Could you check a few things on this drawing? It's one solid part, dimensions in mm from its lowest x, y, z. A direction names the side the tool comes from. Round coordinates to 2 decimals unless told otherwise and drop trailing zeros. Loops run counter-clockwise (first coordinate to the right, second up) from the corner with the lowest first, then second, coordinate; pieces in that order, holes last. Notation, with made-up numbers: (-20, 21.5) -> (39, 21.5) arc R15 cw to (39, 43.5) -> close; hole circle Ø4 at (-14.75, 38). An arc over 180 degrees is marked (long way). Put each result on its own line as item: value. Start each with the question number.
1. Imagine slicing it at B-B, the plane z = 3. Please give me the cut outline in (x, y), and give its area (3 significant figures).
2. Imagine slicing it at A-A, the plane x = 11.1. Please give me the cut outline in (y, z).
3. I need wall thicknesses on line 1 (Y direction, x = 11.1, z = 3); line 2 (Y direction, x = 11.1, z = 7); line 3 (Z direction, x = 13.25, y = 20.75). Which ranges of each line are inside material? Lowest first, please. Write a range as [from, to].
4. Imagine slicing it at C-C, the plane y = 13.5. Please give me the cut outline in (x, z).
5. Imagine slicing it at D-D, the plane x = 19.1. Please give me the cut outline in (y, z), and give its area (3 significant figures).
6. I'm going to push flat-ended pins straight in: P1, Ø4, axis at x = 3.1, y = 11.1, coming from the -Z side; P2, Ø4, axis at x = 11.1, y = 3.1, coming from the +Z side; P3, Ø1, axis at x = 7.5, z = 13.5, coming from the -Y side. Where does each tip first touch, or does it pass through?
7. If we mould it in two halves opening along Y, with no side actions, what happens to the marked faces 1, 2 and 3? For each: pulls with the +Y half, pulls with the -Y half, needs draft (parallel to the pull), parting line crosses it, or undercut.
8. Which directions (+Z, -Z, +X, -X, +Y, -Y) give clear straight access to the entire face, cutting with the end or side of a thin tool? Please do the marked faces 4, 5 and 6.
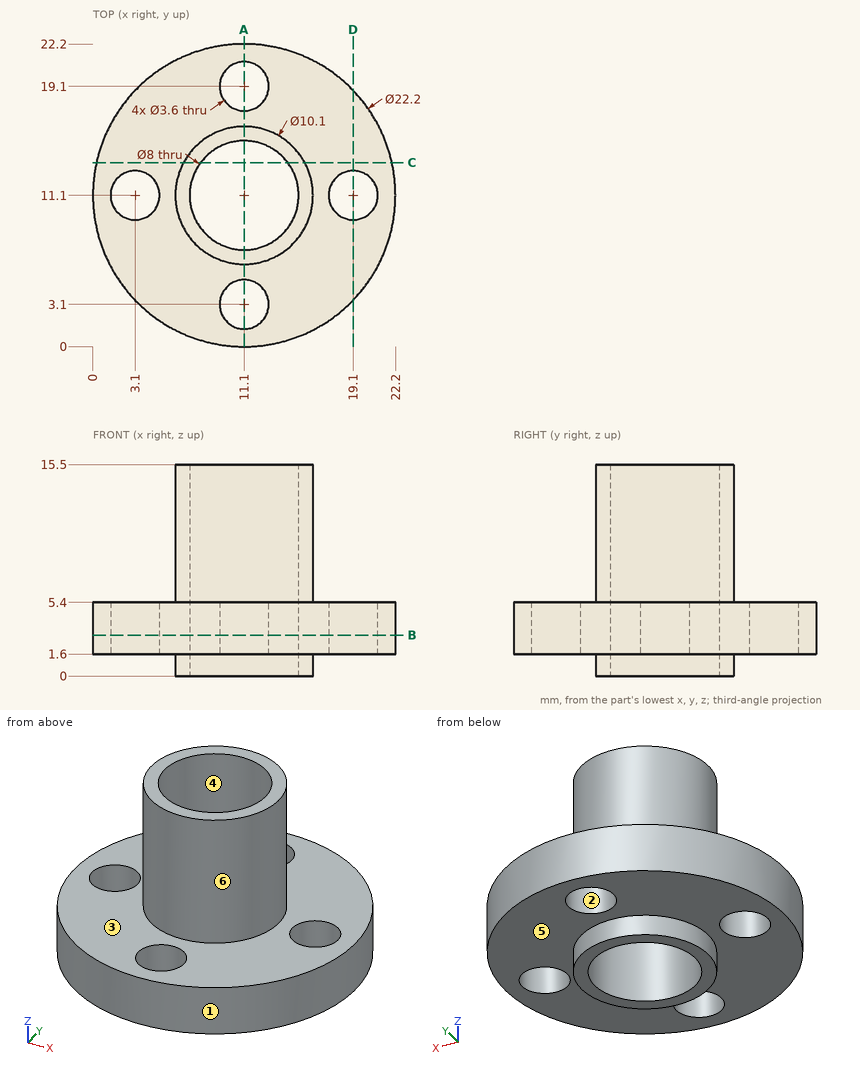
Entries:
1. outline: circle Ø22.2 at (11.1, 11.1); hole circle Ø3.6 at (3.1, 11.1); hole circle Ø8 at (11.1, 11.1); hole circle Ø3.6 at (11.1, 3.1); hole circle Ø3.6 at (11.1, 19.1); hole circle Ø3.6 at (19.1, 11.1)
1. area: 296 mm^2
2. outline: (0, 1.6) -> (1.3, 1.6) -> (1.3, 5.4) -> (0, 5.4) -> close; (4.9, 1.6) -> (6.05, 1.6) -> (6.05, 0) -> (7.1, 0) -> (7.1, 15.5) -> (6.05, 15.5) -> (6.05, 5.4) -> (4.9, 5.4) -> close; (15.1, 0) -> (16.15, 0) -> (16.15, 1.6) -> (17.3, 1.6) -> (17.3, 5.4) -> (16.15, 5.4) -> (16.15, 15.5) -> (15.1, 15.5) -> close; (20.9, 1.6) -> (22.2, 1.6) -> (22.2, 5.4) -> (20.9, 5.4) -> close
3. line 1: [0, 1.3], [4.9, 7.1], [15.1, 17.3], [20.9, 22.2]
3. line 2: [6.05, 7.1], [15.1, 16.15]
3. line 3: [1.6, 5.4]
4. outline: (0.26, 1.6) -> (6.66, 1.6) -> (6.66, 0) -> (7.9, 0) -> (7.9, 15.5) -> (6.66, 15.5) -> (6.66, 5.4) -> (0.26, 5.4) -> close; (14.3, 0) -> (15.54, 0) -> (15.54, 1.6) -> (21.94, 1.6) -> (21.94, 5.4) -> (15.54, 5.4) -> (15.54, 15.5) -> (14.3, 15.5) -> close
5. outline: (3.41, 1.6) -> (9.3, 1.6) -> (9.3, 5.4) -> (3.41, 5.4) -> close; (12.9, 1.6) -> (18.79, 1.6) -> (18.79, 5.4) -> (12.9, 5.4) -> close
5. area: 44.8 mm^2
6. P1: z = 1.6
6. P2: z = 5.4
6. P3: y = 7.11
7. face 1: parting line crosses it
7. face 2: undercut
7. face 3: needs draft
8. face 4: +Z, -Z
8. face 5: -Z
8. face 6: +Z
